```python
from build123d import *

# Parameters (mm, degrees)
SKETCH1_W           = 77
SKETCH1_H           = 165
BOSS_EXTRUDE2_DEPTH = 100
SKETCH4_W           = 67
SKETCH4_H           = 155
CUT_EXTRUDE1_DEPTH  = 95
SKETCH7_W           = 165
SKETCH7_H           = 100
BOSS_EXTRUDE4_DEPTH = 2.5
SKETCH5_W           = 108
SKETCH5_H           = 85
CUT_EXTRUDE2_DEPTH  = 2.5
CUT_EXTRUDE3_REACH  = 152.782
SKETCH9_R           = 2.475
CUT_EXTRUDE4_DEPTH  = 198.24603925
SKETCH11_W          = 165
SKETCH11_H          = 5
BOSS_EXTRUDE5_DEPTH = 30
SKETCH12_R          = 3.775
CUT_EXTRUDE5_DEPTH  = 144.260252687
RIB2_REACH          = 164.054
SKETCH17_WALL_W     = 378.24664849
SKETCH17_WALL_H     = 7
RIB3_REACH          = 195.398
SKETCH18_WALL_W     = 440.934996724
SKETCH18_WALL_H     = 7
RIB5_REACH          = 195.398
SKETCH20_WALL_W     = 440.934996724
SKETCH20_WALL_H     = 7
RIB6_REACH          = 164.054
SKETCH19_WALL_W     = 378.24664849
SKETCH19_WALL_H     = 7
SKETCH21_W          = 108
SKETCH21_H          = 15
BOSS_EXTRUDE6_DEPTH = 13
CUT_EXTRUDE6_REACH  = 168.056
SKETCH23_W          = 8
SKETCH23_H          = 10
SKETCH24_W          = 22.8
SKETCH24_H          = 31
BOSS_EXTRUDE7_DEPTH = 18
CHAMFER1_SIZE       = 2
CHAMFER1_SIZE2      = 3.464101615
CHAMFER2_SIZE       = 2
CHAMFER2_SIZE2      = 3.464101615
SKETCH25_W          = 9
SKETCH25_H          = 13.8
CUT_EXTRUDE7_DEPTH  = 26
CUT_EXTRUDE8_REACH  = 141.995
SKETCH26_R          = 3.775
CUT_EXTRUDE10_REACH = 164.211
SKETCH28_R          = 1.6
CHAMFER3_SIZE       = 2
CHAMFER4_SIZE       = 2
CHAMFER5_SIZE       = 2
CHAMFER6_SIZE       = 2
CUT_EXTRUDE11_REACH = 132.857
SKETCH29_W          = 13
SKETCH29_H          = 8.959672406


with BuildPart() as part:
    # Sketch1 → Boss-Extrude2 (new body)
    with BuildSketch(Plane(origin=(0, 0, 0), x_dir=(1, 0, 0), z_dir=(0, 1, 0))):
        Rectangle(SKETCH1_W, SKETCH1_H)
    extrude(amount=BOSS_EXTRUDE2_DEPTH)

    # Sketch4 → Cut-Extrude1 (cut)
    with BuildSketch(Plane(origin=(0, 100, 0), x_dir=(1, 0, 0), z_dir=(0, 1, 0))):
        Rectangle(SKETCH4_W, SKETCH4_H)
    extrude(amount=-CUT_EXTRUDE1_DEPTH, mode=Mode.SUBTRACT)

    # Sketch7 → Boss-Extrude4 (add)
    with BuildSketch(Plane.ZY.offset(38.5)):
        with Locations((0, 50)):
            Rectangle(SKETCH7_W, SKETCH7_H)
    extrude(amount=BOSS_EXTRUDE4_DEPTH)

    # Sketch5 → Cut-Extrude2 (cut)
    with BuildSketch(Plane.ZY.offset(38.5)):
        with Locations((-23, 85.5)):
            Rectangle(SKETCH5_W, SKETCH5_H)
    extrude(amount=CUT_EXTRUDE2_DEPTH, mode=Mode.SUBTRACT)

    # Sketch9 → Cut-Extrude3 (cut, up to next)
    with BuildSketch(Plane.ZY.offset(38.5), mode=Mode.PRIVATE) as cut_extrude3_sk1:
        with Locations((-71.5, 85.5)):
            Circle(SKETCH9_R)
    cut_extrude3_tool1 = extrude(cut_extrude3_sk1.sketch, amount=-CUT_EXTRUDE3_REACH, mode=Mode.PRIVATE) & part.part
    # Sketch9 → Cut-Extrude3 (cut, up to next)
    with BuildSketch(Plane.ZY.offset(38.5), mode=Mode.PRIVATE) as cut_extrude3_sk2:
        with Locations((25.5, 85.5)):
            Circle(SKETCH9_R)
    cut_extrude3_tool2 = extrude(cut_extrude3_sk2.sketch, amount=-CUT_EXTRUDE3_REACH, mode=Mode.PRIVATE) & part.part
    add(cut_extrude3_tool1.solids().sort_by_distance((-38.5, 85.5, -71.5))[0], mode=Mode.SUBTRACT)
    add(cut_extrude3_tool2.solids().sort_by_distance((-38.5, 85.5, 25.5))[0], mode=Mode.SUBTRACT)

    # Sketch10 → Cut-Extrude4 (cut, through all)
    with BuildSketch(Plane.XY.offset(82.5)):
        with BuildLine():
            Line((12.62916064, 100), (12.62916064, 62.639075144))
            ThreePointArc((12.62916064, 62.639075144), (0, 50.009914504), (-12.62916064, 62.639075144))
            Line((-12.62916064, 62.639075144), (-12.62916064, 100))
            ThreePointArc((-12.62916064, 100), (0, 112.62916064), (12.62916064, 100))
        make_face()
    extrude(amount=-CUT_EXTRUDE4_DEPTH, mode=Mode.SUBTRACT)

    # Sketch11 → Boss-Extrude5 (add)
    with BuildSketch(Plane(origin=(38.5, 0, 0), x_dir=(0, 0, -1), z_dir=(1, 0, 0))):
        with Locations((0, 2.5)):
            Rectangle(SKETCH11_W, SKETCH11_H)
    extrude(amount=BOSS_EXTRUDE5_DEPTH)

    # Sketch12 → Cut-Extrude5 (cut, through all)
    with BuildSketch(Plane(origin=(0, 5, 0), x_dir=(1, 0, 0), z_dir=(0, 1, 0))):
        with Locations(Location((60, 50.12, 0), (0, 0, 270))):
            Circle(SKETCH12_R)
        with Locations(Location((60, 0, 0), (0, 0, 270))):
            Circle(SKETCH12_R)
        with Locations(Location((60, -50.12, 0), (0, 0, 270))):
            Circle(SKETCH12_R)
    extrude(amount=-CUT_EXTRUDE5_DEPTH, mode=Mode.SUBTRACT)

    # Sketch17 wall → Rib2 (add, up to next)
    with BuildSketch(Plane(origin=(49.25, 28.75, 25.06), x_dir=(-0.412357398674, 0.911022159861, 0), z_dir=(-0.911022159861, -0.412357398674, 0)), mode=Mode.PRIVATE) as rib2_sk1:
        Rectangle(SKETCH17_WALL_W, SKETCH17_WALL_H)
    rib2_tool1 = extrude(rib2_sk1.sketch, amount=RIB2_REACH, mode=Mode.PRIVATE) - part.part
    add(rib2_tool1.solids().sort_by_distance((49.25, 28.75, 25.06))[0])

    # Sketch18 wall → Rib3 (add, up to next)
    with BuildSketch(Plane(origin=(49.25, 28.75, 68.2), x_dir=(0.412357398674, -0.911022159861, 0), z_dir=(0.911022159861, 0.412357398674, 0)), mode=Mode.PRIVATE) as rib3_sk1:
        Rectangle(SKETCH18_WALL_W, SKETCH18_WALL_H)
    rib3_tool1 = extrude(rib3_sk1.sketch, amount=-RIB3_REACH, mode=Mode.PRIVATE) - part.part
    add(rib3_tool1.solids().sort_by_distance((49.25, 28.75, 68.2))[0])

    # Sketch20 wall → Rib5 (add, up to next)
    with BuildSketch(Plane(origin=(49.25, 28.75, -68.2), x_dir=(-0.412357398674, 0.911022159861, 0), z_dir=(-0.911022159861, -0.412357398674, 0)), mode=Mode.PRIVATE) as rib5_sk1:
        Rectangle(SKETCH20_WALL_W, SKETCH20_WALL_H)
    rib5_tool1 = extrude(rib5_sk1.sketch, amount=RIB5_REACH, mode=Mode.PRIVATE) - part.part
    add(rib5_tool1.solids().sort_by_distance((49.25, 28.75, -68.2))[0])

    # Sketch19 wall → Rib6 (add, up to next)
    with BuildSketch(Plane(origin=(49.25, 28.75, -25.06), x_dir=(-0.412357398674, 0.911022159861, 0), z_dir=(-0.911022159861, -0.412357398674, 0)), mode=Mode.PRIVATE) as rib6_sk1:
        Rectangle(SKETCH19_WALL_W, SKETCH19_WALL_H)
    rib6_tool1 = extrude(rib6_sk1.sketch, amount=RIB6_REACH, mode=Mode.PRIVATE) - part.part
    add(rib6_tool1.solids().sort_by_distance((49.25, 28.75, -25.06))[0])

    # Sketch21 → Boss-Extrude6 (add)
    with BuildSketch(Plane.ZY.offset(41)):
        with Locations((-23, 17.5)):
            Rectangle(SKETCH21_W, SKETCH21_H)
    extrude(amount=BOSS_EXTRUDE6_DEPTH)

    # Sketch23 → Cut-Extrude6 (cut, up to next)
    with BuildSketch(Plane.XY.offset(31), mode=Mode.PRIVATE) as cut_extrude6_sk1:
        with Locations((-45, 15)):
            Rectangle(SKETCH23_W, SKETCH23_H)
    cut_extrude6_tool1 = extrude(cut_extrude6_sk1.sketch, amount=-CUT_EXTRUDE6_REACH, mode=Mode.PRIVATE) & part.part
    add(cut_extrude6_tool1.solids().sort_by_distance((-45, 15, 31))[0], mode=Mode.SUBTRACT)

    # Sketch24 → Boss-Extrude7 (add)
    with BuildSketch(Plane.ZY.offset(41)):
        with Locations((53.4, 79.5)):
            Rectangle(SKETCH24_W, SKETCH24_H)
    extrude(amount=BOSS_EXTRUDE7_DEPTH)

    # Chamfer1
    chamfer1_edges = [part.edges().sort_by_distance(p)[0] for p in [
        (-33.5, 85.5, 23.025),
    ]]
    chamfer1_side = [part.faces().sort_by_distance(p)[0] for p in [
        (-33.5, 52.413518032, 0.060275311),
    ]]
    chamfer(chamfer1_edges, length=CHAMFER1_SIZE, length2=CHAMFER1_SIZE2, reference=chamfer1_side[0])

    # Chamfer2
    chamfer2_edges = [part.edges().sort_by_distance(p)[0] for p in [
        (-33.5, 85.5, -73.975),
    ]]
    chamfer2_side = [part.faces().sort_by_distance(p)[0] for p in [
        (-33.5, 52.31484696, -0.015591471),
    ]]
    chamfer(chamfer2_edges, length=CHAMFER2_SIZE, length2=CHAMFER2_SIZE2, reference=chamfer2_side[0])

    # Sketch25 → Cut-Extrude7 (cut)
    with BuildSketch(Plane.XZ.offset(-64)):
        with Locations((-50, 53.4)):
            Rectangle(SKETCH25_W, SKETCH25_H)
    extrude(amount=-CUT_EXTRUDE7_DEPTH, mode=Mode.SUBTRACT)

    # Sketch26 → Cut-Extrude8 (cut, up to next)
    with BuildSketch(Plane.XZ.offset(-90), mode=Mode.PRIVATE) as cut_extrude8_sk1:
        with Locations(Location((-50, 53.4, 0), (0, 0, 270))):
            Circle(SKETCH26_R)
    cut_extrude8_tool1 = extrude(cut_extrude8_sk1.sketch, amount=-CUT_EXTRUDE8_REACH, mode=Mode.PRIVATE) & part.part
    add(cut_extrude8_tool1.solids().sort_by_distance((-50, 90, 53.4))[0], mode=Mode.SUBTRACT)

    # Sketch28 → Cut-Extrude10 (cut, up to next)
    with BuildSketch(Plane(origin=(38.5, 0, 0), x_dir=(0, 0, -1), z_dir=(1, 0, 0)), mode=Mode.PRIVATE) as cut_extrude10_sk1:
        with Locations((-15, 96)):
            Circle(SKETCH28_R)
    cut_extrude10_tool1 = extrude(cut_extrude10_sk1.sketch, amount=-CUT_EXTRUDE10_REACH, mode=Mode.PRIVATE) & part.part
    # Sketch28 → Cut-Extrude10 (cut, up to next)
    with BuildSketch(Plane(origin=(38.5, 0, 0), x_dir=(0, 0, -1), z_dir=(1, 0, 0)), mode=Mode.PRIVATE) as cut_extrude10_sk2:
        with Locations((-15, 54.648)):
            Circle(SKETCH28_R)
    cut_extrude10_tool2 = extrude(cut_extrude10_sk2.sketch, amount=-CUT_EXTRUDE10_REACH, mode=Mode.PRIVATE) & part.part
    # Sketch28 → Cut-Extrude10 (cut, up to next)
    with BuildSketch(Plane(origin=(38.5, 0, 0), x_dir=(0, 0, -1), z_dir=(1, 0, 0)), mode=Mode.PRIVATE) as cut_extrude10_sk3:
        with Locations((51.5, 96)):
            Circle(SKETCH28_R)
    cut_extrude10_tool3 = extrude(cut_extrude10_sk3.sketch, amount=-CUT_EXTRUDE10_REACH, mode=Mode.PRIVATE) & part.part
    # Sketch28 → Cut-Extrude10 (cut, up to next)
    with BuildSketch(Plane(origin=(38.5, 0, 0), x_dir=(0, 0, -1), z_dir=(1, 0, 0)), mode=Mode.PRIVATE) as cut_extrude10_sk4:
        with Locations((51.5, 54.648)):
            Circle(SKETCH28_R)
    cut_extrude10_tool4 = extrude(cut_extrude10_sk4.sketch, amount=-CUT_EXTRUDE10_REACH, mode=Mode.PRIVATE) & part.part
    add(cut_extrude10_tool1.solids().sort_by_distance((38.5, 96, 15))[0], mode=Mode.SUBTRACT)
    add(cut_extrude10_tool2.solids().sort_by_distance((38.5, 54.648, 15))[0], mode=Mode.SUBTRACT)
    add(cut_extrude10_tool3.solids().sort_by_distance((38.5, 96, -51.5))[0], mode=Mode.SUBTRACT)
    add(cut_extrude10_tool4.solids().sort_by_distance((38.5, 54.648, -51.5))[0], mode=Mode.SUBTRACT)

    # Chamfer3
    chamfer3_edges = [part.edges().sort_by_distance(p)[0] for p in [
        (33.5, 96, 16.6),
    ]]
    chamfer(chamfer3_edges, length=CHAMFER3_SIZE)

    # Chamfer4
    chamfer4_edges = [part.edges().sort_by_distance(p)[0] for p in [
        (33.5, 54.648, 16.6),
    ]]
    chamfer(chamfer4_edges, length=CHAMFER4_SIZE)

    # Chamfer5
    chamfer5_edges = [part.edges().sort_by_distance(p)[0] for p in [
        (33.5, 96, -49.9),
    ]]
    chamfer(chamfer5_edges, length=CHAMFER5_SIZE)

    # Chamfer6
    chamfer6_edges = [part.edges().sort_by_distance(p)[0] for p in [
        (33.5, 54.648, -49.9),
    ]]
    chamfer(chamfer6_edges, length=CHAMFER6_SIZE)

    # Sketch29 → Cut-Extrude11 (cut, up to next)
    with BuildSketch(Plane(origin=(0, 25, 0), x_dir=(1, 0, 0), z_dir=(0, 1, 0)), mode=Mode.PRIVATE) as cut_extrude11_sk1:
        with Locations((-47.5, 18.520163797)):
            Rectangle(SKETCH29_W, SKETCH29_H)
    cut_extrude11_tool1 = extrude(cut_extrude11_sk1.sketch, amount=-CUT_EXTRUDE11_REACH, mode=Mode.PRIVATE) & part.part
    add(cut_extrude11_tool1.solids().sort_by_distance((-47.5, 25, -18.520164))[0], mode=Mode.SUBTRACT)


solid = part.part
```
Design review of the part built by this model. Coordinates are the model's own, in mm. A direction names the side the tool comes from. Give positions to 0.01 mm unless a question says otherwise; leave off trailing zeros. Write each loop counter-clockwise with the first axis right and the second up, starting at its lowest first coordinate (ties: lowest second). Pieces come first, ordered by that corner, then holes. Notation, with made-up numbers: (-13.5, -38.75) - (-3.5, -38.75) arc R9 ccw to (-3.5, -31.75) - close; hole circle Ø1 at (76.25, 80.25). An arc over 180 degrees is marked (long way). Return JSON: item names as keys, results as strings. Group by question number.
(1) To check wall thickness, follow probe 1 along X at (y, z) = (92.3, 53.4) (3 decimals); probe 2 along Z at (x, y) = (41, 15.5); probe 3 along X at (y, z) = (42.5, 67). State the ranges of each line that lie inside material, in increasing order.
(2) We need section A-A, the plane y = 74. Give the boundary of the cut face in (x, z).
(3) Insertion check: pin 1 (3 mm diameter, centred on y = 82.5, z = -24.5, fed in from +X); pin 2 (8 mm diameter, centred on y = 85.5, z = -71.5, fed in from -X); pin 3 (4 mm diameter, centred on x = -44.5, z = 9.5, fed in from +Y). Each pin has a flat end and moves straight along its axis. Give the tip position at first contact, or say it passes through.
(4) We need section D-D, the plane x = 0. Give the boundary of the cut face in (y, z), then the cut area to 3 significant figures.
(5) We need section C-C, the plane y = 85.5. Give the number of separate pieces and of enclosed holes in the cut face, then the cut area to 3 significant figures.
(6) Machinability: for faces 4 (the flat face through (45, 20, -71.7)), 5 (the conical face through (-36.8, 88.05, -71.83)), 6 (the flat face through (45, 20, -28.56)), which of the approach directions +Z, -Z, +X, -X, +Y, -Y give a long, thin tool a straight path to every point of the face, cutting with its end or side? Answer none if there is none.
(7) We need section B-B, the plane z = 25.5. Give the boundary of the cut face in (x, y) (3 decimals).
(8) Mouldability with a two-part tool opening along X and no side actions: class faces 1 (the conical face through (-36.8, 88.05, 25.17)), 2 (the flat face through (-59, 80, 53)), 3 (the flat face through (-47, 25, 8)) as +X half, -X half, draft (parallel to the pull), parting line (faces both ways), or undercut.
Reported:
{
 "1": {"probe 1": "x = -59 to -53.775, -46.225 to -33.5, 33.5 to 38.5", "probe 2": "z = -71.7 to -64.7, -28.56 to -21.56, 21.56 to 28.56, 64.7 to 71.7", "probe 3": "x = -41 to -33.5, 33.5 to 43.03"},
 "2": {"outline": "(-59, 42) - (-41, 42) - (-41, 31) - (-38.5, 31) - (-38.5, -77) - (-41, -77) - (-41, -82.5) - (-12.63, -82.5) - (-12.63, -77.5) - (-33.5, -77.5) - (-33.5, 77.5) - (-12.63, 77.5) - (-12.63, 82.5) - (-41, 82.5) - (-41, 64.8) - (-59, 64.8) - close; (12.63, -82.5) - (38.5, -82.5) - (38.5, 82.5) - (12.63, 82.5) - (12.63, 77.5) - (33.5, 77.5) - (33.5, -77.5) - (12.63, -77.5) - close; hole (-54.5, 46.5) - (-45.5, 46.5) - (-45.5, 60.3) - (-54.5, 60.3) - close"},
 "3": {"pin 1": "stops at x = 38.5", "pin 2": "stops at x = -38.5", "pin 3": "stops at y = 25"},
 "4": {"outline": "(0, -82.5) - (50.01, -82.5) - (50.01, -77.5) - (5, -77.5) - (5, 77.5) - (50.01, 77.5) - (50.01, 82.5) - (0, 82.5) - close", "area": "1,280 mm2"},
 "5": {"separate pieces": "4", "enclosed holes": "1", "area": "2,430 mm2"},
 "6": {"face 4": "-Z, +X, +Y", "face 5": "none", "face 6": "+X, +Y"},
 "7": {"outline": "(-54, 10) - (-49, 10) - (-49, 20) - (-41, 20) - (-41, 0) - (68.5, 0) - (68.5, 5) - (60, 5) - (38.5, 52.5) - (38.5, 100) - (33.5, 100) - (33.5, 5) - (-33.5, 5) - (-33.5, 81.025) - (-36.964, 83.025) - (-38.5, 83.025) - (-38.5, 43) - (-41, 43) - (-41, 25) - (-54, 25) - close; (-38.5, 87.975) - (-36.964, 87.975) - (-33.5, 89.975) - (-33.5, 100) - (-38.5, 100) - close"},
 "8": {"face 1": "undercut", "face 2": "-X half", "face 3": "draft"}
}
